Geometry: final body of the model. Coordinates: model frame, mm. A direction names the side the tool comes from. Coordinates: 2 decimals unless noted, no trailing zeros. Order: outer loops, then holes, each group sorted by start corner. A loop starts at its lowest first (then second) coordinate and runs counter-clockwise, first axis right, second up. Notation, with made-up numbers: (-30.75, 20) - (-22.75, 20) arc R15 cw to (-22.75, 28) - close; hole circle Ø10 at (-31.5, -14.5). An arc over 180 degrees is marked (long way). Use a Markdown table: item, result. Add a question column.
```python
from build123d import *

# Parameters (mm, degrees)
SKETCH1_W               = 30
SKETCH1_H               = 25
BOSS_EXTRUDE1_DEPTH     = 5
BOSS_EXTRUDE6_START     = -5
BOSS_EXTRUDE6_OUTLINE_W = 5
BOSS_EXTRUDE6_OUTLINE_H = 13
BOSS_EXTRUDE6_DEPTH     = 5
SKETCH5_R               = 35.5
CUT_EXTRUDE1_DEPTH      = 31


# Read off the part's stored shape, not the designer's step: Boss-Extrude6
with BuildPart() as part:
    # Sketch1 → Boss-Extrude1 (new body)
    with BuildSketch(Plane.XY):
        with Locations((15, 12.5)):
            Rectangle(SKETCH1_W, SKETCH1_H)
    extrude(amount=BOSS_EXTRUDE1_DEPTH)

    # Boss-Extrude6 outline → Boss-Extrude6 (cut)
    with BuildSketch(Plane.XY.offset(5).offset(BOSS_EXTRUDE6_START)):
        with Locations((15, 18.5)):
            Rectangle(BOSS_EXTRUDE6_OUTLINE_W, BOSS_EXTRUDE6_OUTLINE_H)
    extrude(amount=BOSS_EXTRUDE6_DEPTH, mode=Mode.SUBTRACT)

    # Sketch5 → Cut-Extrude1 (cut)
    with BuildSketch(Plane.XY.offset(5)):
        with Locations((15, 58)):
            Circle(SKETCH5_R)
    extrude(amount=-CUT_EXTRUDE1_DEPTH, mode=Mode.SUBTRACT)


solid = part.part
```
1) Draft query along X for faces 3 (the flat face through (0, 12, 2)), 4 (the flat face through (29, 25, 2)), 5 (the flat face through (15, 12, 2)), 6 (the flat face through (12.5, 17, 2)). Return one class per face: released by +X, released by -X, zero draft, split by the parting line, or undercut.
2) Access query for faces 1 (the flat face through (15, 10, 5)), 2 (the cylindrical face through (22.81, 23.37, 2.54)). Directions: +Z, -Z, +X, -X, +Y, -Y. A direction counts if a zero-diameter tool reaches every point of the face in a straight line with its end or side. Return the directions, or none.
3) Section query D-D (x = 10.5). Return the cut outline in (y, z), and give its area (3 significant figures).
4) Line query: line 1 (X direction, y = 15, z = 1.1); line 2 (Y direction, x = 13, z = 1.45); line 3 (Y direction, x = 18, z = 3.15). Output: solid intervals per line, ascending. Write a range as from..to.
5) Section query B-B (z = 3.65). Return the cut outline in (x, y), and give its area (3 significant figures).
6) First-contact query: pin 1 (5 mm diameter, centred on x = 24.5, y = 12.5, fed in from -Z); pin 2 (1.5 mm diameter, centred on x = 15, z = 2.5, fed in from +Y). Flat tips, straight axial feed; report the tip coordinate or a pass-through.
7) Section query A-A (y = 19). Return the cut outline in (x, z), and give its area (3 significant figures).
8) Section query C-C (x = 14.75). Return the cut outline in (y, z).
From the geometry:
| question | item | result |
|---|---|---|
| 1 | face 3 | released by -X |
| 1 | face 4 | zero draft |
| 1 | face 5 | undercut |
| 1 | face 6 | undercut |
| 2 | face 1 | +Z, +X, -X, +Y, -Y |
| 2 | face 2 | +Z, -Z, +Y |
| 3 | outline | (0, 0) - (22.79, 0) - (22.79, 5) - (0, 5) - close |
| 3 | area | 114 mm^2 |
| 4 | line 1 | x = 0..12.5, 17.5..30 |
| 4 | line 2 | y = 0..12 |
| 4 | line 3 | y = 0..22.63 |
| 5 | outline | (0, 0) - (30, 0) - (30, 25) - (28.09, 25) arc R35.5 cw to (17.5, 22.59) - (17.5, 12) - (12.5, 12) - (12.5, 22.59) arc R35.5 cw to (1.91, 25) - (0, 25) - close |
| 5 | area | 653 mm^2 |
| 6 | pin 1 | stops at z = 0 |
| 6 | pin 2 | stops at y = 12 |
| 7 | outline | (0, 0) - (12.5, 0) - (12.5, 5) - (0, 5) - close; (17.5, 0) - (30, 0) - (30, 5) - (17.5, 5) - close |
| 7 | area | 125 mm^2 |
| 8 | outline | (0, 0) - (12, 0) - (12, 5) - (0, 5) - close |
